from build123d import *

# Parameters (mm, degrees)
F0_W           = 100
F0_H           = 100
F1_DEPTH       = 25
F2_W           = 40
F2_H           = 40
F3_DEPTH       = 25
F5_D           = 5
F5_CBORE_D     = 10
F5_CBORE_DEPTH = 5
F7_D           = 5.5


with BuildPart() as f1:
    # F0 (on Front) → F1 (new body)
    with BuildSketch(Plane.XZ):
        with Locations((50, 50)):
            Rectangle(F0_W, F0_H)
    extrude(amount=F1_DEPTH)

    # F2 (on face) → F3 (cut)
    with BuildSketch(Plane.XZ.offset(25)):
        with Locations((50, 50)):
            Rectangle(F2_W, F2_H)
    extrude(amount=-F3_DEPTH, mode=Mode.SUBTRACT)

    # F5 (through all)
    with Locations(Plane.XZ.offset(25)):
        with Locations((90, 90)):
            CounterBoreHole(F5_D / 2, F5_CBORE_D / 2, F5_CBORE_DEPTH)

    # F7 (through all)
    with Locations(Plane.XZ.offset(25)):
        with Locations((15, 15)):
            Hole(F7_D / 2)


solid = f1.part
Input: part model. Units: mm. Frame: model coordinates. A direction names the side the tool comes from. Give positions to 0.01 mm unless a question says otherwise; leave off trailing zeros. Order: outer loops, then holes, each group sorted by start corner. A loop starts at its lowest first (then second) coordinate and runs counter-clockwise, first axis right, second up.
Q1. Section C-C on y = -18.25. Output: boundary loops of the cut face in (x, z).
Checked values:
outline: (0, 0) - (100, 0) - (100, 100) - (0, 100) - close; hole circle Ø5.5 at (15, 15); hole (30, 30) - (70, 30) - (70, 70) - (30, 70) - close; hole circle Ø5 at (90, 90)
Q2. Contact query for a flat-ended pin moving along its axis: pin 1 Ø8 at (x, z) = (90, 90) entering from +Y. Output: stop coordinate, or through.
Checked values:
pin 1: stops at y = 0
Q3. Set-up query: faces 5 (the flat face through (100, -12, 49)), 6 (the flat face through (30, -13, 50)), 7 (the cylindrical face through (94.619, -22.535, 88.085)). Return all of +Z, -Z, +X, -X, +Y, -Y with unobstructed straight access to the full face (end or side cutting, diameter ignored); none if empty.
Checked values:
face 5: +Z, -Z, +X, +Y, -Y
face 6: +Y, -Y
face 7: -Y
Q4. Draft query along Z for faces 1 (the flat face through (49, -25, 73)), 2 (the flat face through (49, -12, 100)), 3 (the flat face through (49, -12, 0)), 4 (the cylindrical face through (90.33, -9.86, 92.48)). Return one class per face: +Z half, -Z half, draft (parallel to the pull), parting line (faces both ways), or undercut.
Checked values:
face 1: draft
face 2: +Z half
face 3: -Z half
face 4: undercut
Q5. Section B-B on x = 39. Output: boundary loops of the cut face in (y, z), and give its area (3 significant figures).
Checked values:
outline: (-25, 0) - (0, 0) - (0, 30) - (-25, 30) - close; (-25, 70) - (0, 70) - (0, 100) - (-25, 100) - close
area: 1,500 mm2
Q6. Section A-A on z = 90. Output: boundary loops of the cut face in (x, y).
Checked values:
outline: (0, -25) - (85, -25) - (85, -20) - (87.5, -20) - (87.5, 0) - (0, 0) - close; (92.5, -20) - (95, -20) - (95, -25) - (100, -25) - (100, 0) - (92.5, 0) - close
Q7. Section D-D on z = 40. Output: boundary loops of the cut face in (x, y).
Checked values:
outline: (0, -25) - (30, -25) - (30, 0) - (0, 0) - close; (70, -25) - (100, -25) - (100, 0) - (70, 0) - close
Q8. Ray query, probe 1 along Z at (x, y) = (51, -18.25); probe 2 along Z at (x, y) = (90, -23.8). Return the intervals inside material, ascending.
Checked values:
probe 1: z = 0 to 30, 70 to 100
probe 2: z = 0 to 85, 95 to 100
